```python
from build123d import *

# Parameters (mm, degrees)
EXTRUDE_1_DEPTH     = 6
EXTRUDE_2_DEPTH     = 2
CUT_EXTRUDE_1_DEPTH = 0.8


with BuildPart() as part:
    # 草图1 → 凸台-拉伸1 (new body)
    with BuildSketch(Plane.XY):
        Polygon((41.469502686, 98.413945938), (1.599546065, 58.543989317), (1.599546065, 41.382573206), (41.469502686, 1.512616585), (58.630918797, 1.512616585), (98.500875418, 41.382573206), (98.500875418, 58.543989317), (58.630918797, 98.413945938), align=None)
        Polygon((43.126356936, 94.413945938), (5.599546065, 56.887135068), (5.599546065, 43.039427456), (43.126356936, 5.512616585), (56.974064547, 5.512616585), (94.500875418, 43.039427456), (94.500875418, 56.887135068), (56.974064547, 94.413945938), align=None, mode=Mode.SUBTRACT)
    extrude(amount=-EXTRUDE_1_DEPTH)

    # 草图3 → 凸台-拉伸2 (add)
    with BuildSketch(Plane.XY):
        Polygon((43.126356936, 94.413945938), (5.599546065, 56.887135068), (5.599546065, 43.039427456), (43.126356936, 5.512616585), (56.974064547, 5.512616585), (94.500875418, 43.039427456), (94.500875418, 56.887135068), (56.974064547, 94.413945938), align=None)
    extrude(amount=-EXTRUDE_2_DEPTH)

    # 草图4 → 切除-拉伸1 (cut)
    with BuildSketch(Plane(origin=(0, 0, -2), x_dir=(-1, 0, 0), z_dir=(0, 0, -1))):
        Polygon((-94.500875418, 56.887135068), (-94.500875418, 51.791965689), (-45.081351484, 51.791965689), (-31.918303141, 64.736865353), (-43.433956755, 76.502141218), (-74.885869267, 76.502141218), align=None)
        Polygon((-56.974064547, 94.413945938), (-63.930144523, 87.457865962), (-43.030556381, 87.457865962), (-31.044508785, 74.652044034), (-35.091931028, 70.863720572), (-33.339917404, 68.991879642), (-17.704290639, 68.991879642), (-43.126356936, 94.413945938), align=None)
        Polygon((-54.339287077, 23.853509746), (-24.785463775, 23.853509746), (-5.599546065, 43.039427456), (-5.599546065, 48.49814838), (-56.346633262, 48.49814838), (-67.681954242, 36.947928988), align=None)
        Polygon((-66.584102119, 31.663565611), (-83.125013573, 31.663565611), (-56.974064547, 5.512616585), (-43.126356936, 5.512616585), (-35.72811274, 12.910860781), (-57.7675839, 12.910860781), (-69.485376795, 25.556943884), (-64.977324173, 30.052221354), align=None)
    extrude(amount=-CUT_EXTRUDE_1_DEPTH, mode=Mode.SUBTRACT)


solid = part.part
```
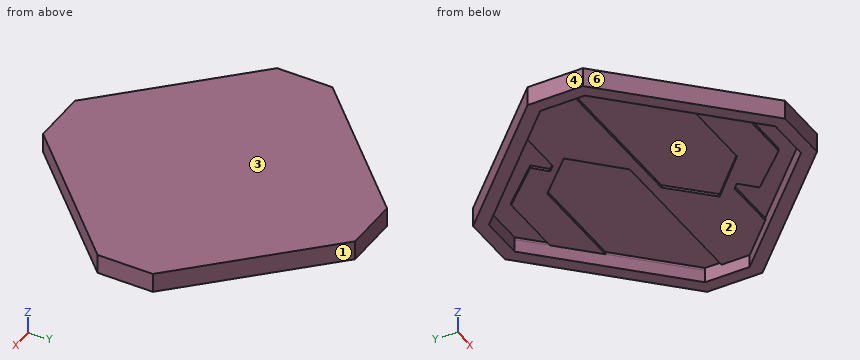
Part model, mm, in its own coordinate system. Face numbers are marked on the shaded views. A direction names the side the tool comes from. Round coordinates to 2 decimals unless told otherwise and drop trailing zeros. Write each loop counter-clockwise with the first axis right and the second up, starting at its lowest first coordinate (ties: lowest second). Pieces come first, ordered by that corner, then holes.
Item 1: Which spindle directions (+Z, -Z, +X, -X, +Y, -Y) get a long thin tool onto all of the face, cutting with end or side? Do the marked faces 5 and 6. Say none if no direction does.
Results:
face 5: -Z
face 6: +Z, -Z, -X, -Y
Item 2: Drop flat-ended pins along their axis: pin 1 Ø1.5 at (y, z) = (71.5, -0.5) entering from +X; pin 2 Ø8 at (x, y) = (55.5, 21) entering from -Z; pin 3 Ø7.5 at (x, y) = (35, 34) entering from -Z; pin 4 Ø3 at (x, y) = (38.5, 77) entering from +Z. Give the stop position or say it passes through.
Results:
pin 1: stops at x = 86.29
pin 2: stops at z = -2
pin 3: stops at z = -1.2
pin 4: stops at z = 0
Item 3: Cut at A-A, the plane z = -4.8. Give the cut face in (x, y).
Results:
outline: (1.6, 41.38) - (41.47, 1.51) - (58.63, 1.51) - (98.5, 41.38) - (98.5, 58.54) - (58.63, 98.41) - (41.47, 98.41) - (1.6, 58.54) - close; hole (5.6, 43.04) - (43.13, 5.51) - (56.97, 5.51) - (94.5, 43.04) - (94.5, 56.89) - (56.97, 94.41) - (43.13, 94.41) - (5.6, 56.89) - close
Item 4: Cut at B-B, the plane x = 8.5. Give the cut face in (y, z), plus the area to 3 significant figures.
Results:
outline: (34.48, -6) - (40.14, -6) - (40.14, -1.2) - (48.5, -1.2) - (48.5, -2) - (59.79, -2) - (59.79, -6) - (65.44, -6) - (65.44, 0) - (34.48, 0) - close
area: 100 mm2
Item 5: Probe L1, parallel to X at y = 55, z = -2.05; L2, parallel to Y at x = 54, z = -4.6; L3, parallel to Y at x = 28, z = -1.7. List the from-to ranges inside material, lowest first.
Results:
L1: x = 1.6 to 5.6, 94.5 to 98.5
L2: y = 1.51 to 5.51, 94.41 to 98.41
L3: y = 14.98 to 23.85, 48.5 to 68.99, 79.29 to 84.94
Item 6: Two-plate mould, pull along X, no slides. Class the marked faces 1, 2, 3 and 4: +X half, -X half, draft (parallel to the pull), parting line (faces both ways), or undercut.
Results:
face 1: +X half
face 2: undercut
face 3: draft
face 4: -X half
Item 7: Cut at C-C, the plane y = 54. Give the cut face in (x, z).
Results:
outline: (1.6, -6) - (5.6, -6) - (5.6, -2) - (42.84, -2) - (42.84, -1.2) - (94.5, -1.2) - (94.5, -6) - (98.5, -6) - (98.5, 0) - (1.6, 0) - close
Item 8: Cut at D-D, the plane x = 61. Give the cut face in (y, z), plus the area to 3 significant figures.
Results:
outline: (3.88, -6) - (9.54, -6) - (9.54, -1.2) - (16.4, -1.2) - (16.4, -2) - (30.39, -2) - (30.39, -1.2) - (43.76, -1.2) - (43.76, -2) - (51.79, -2) - (51.79, -1.2) - (76.5, -1.2) - (76.5, -2) - (87.46, -2) - (87.46, -1.2) - (90.39, -1.2) - (90.39, -6) - (96.04, -6) - (96.04, 0) - (3.88, 0) - close
area: 191 mm2
